Source: three-view drawing plus pictorial views. Frame: mm from the lowest corner of the part. A direction names the side the tool comes from. Round coordinates to 2 decimals unless told otherwise and drop trailing zeros. Loops run counter-clockwise (first coordinate to the right, second up) from the corner with the lowest first, then second, coordinate; pieces in that order, holes last. Notation, with made-up numbers: (-24, 84) -> (22, 84) arc R17 cw to (22, 89) -> close; hole circle Ø10 at (54.25, -39). An arc over 180 degrees is marked (long way). Answer as a JSON object with one key per item and string values. Group by question number.
Item 1: Section query C-C on y = 3.75. Return loops of the section in (x, z), and give its area (3 significant figures).
Item 2: Section query D-D on z = 3. Return loops of the section in (x, y).
Item 3: Section query A-A on x = 2.5. Return loops of the section in (y, z), and give its area (3 significant figures).
Item 4: Pin query (flat end, axial travel): pin 1 (2 mm diameter, centred on y = 1, z = 8, fed in from -X); pin 2 (4 mm diameter, centred on x = 2.5, z = 7, fed in from -Y); pin 3 (0.8 mm diameter, centred on y = 1, z = 6.5, fed in from +X); pin 4 (4 mm diameter, centred on x = 35.5, y = 5, fed in from -Z). Return the tip coordinate at first contact, or that it passes through.
Item 5: Material intervals for line 1 (Z direction, x = 47.5, y = 4.3); line 2 (Z direction, x = 25, y = 3.25); line 3 (X direction, y = 7.25, z = 8), sorted ascending. Write a range as [from, to].
Item 6: Section query B-B on z = 10. Return loops of the section in (x, y).
Item 7: Draft query along Z for the marked faces 1, 2, 3 and 4. Return one class per face: released by +Z, released by -Z, zero draft, split by the parting line, or undercut.
Item 8: Set-up query: the marked faces 5 and 6. Return all of +Z, -Z, +X, -X, +Y, -Y with unobstructed straight access to the full face (end or side cutting, diameter ignored); none if empty.
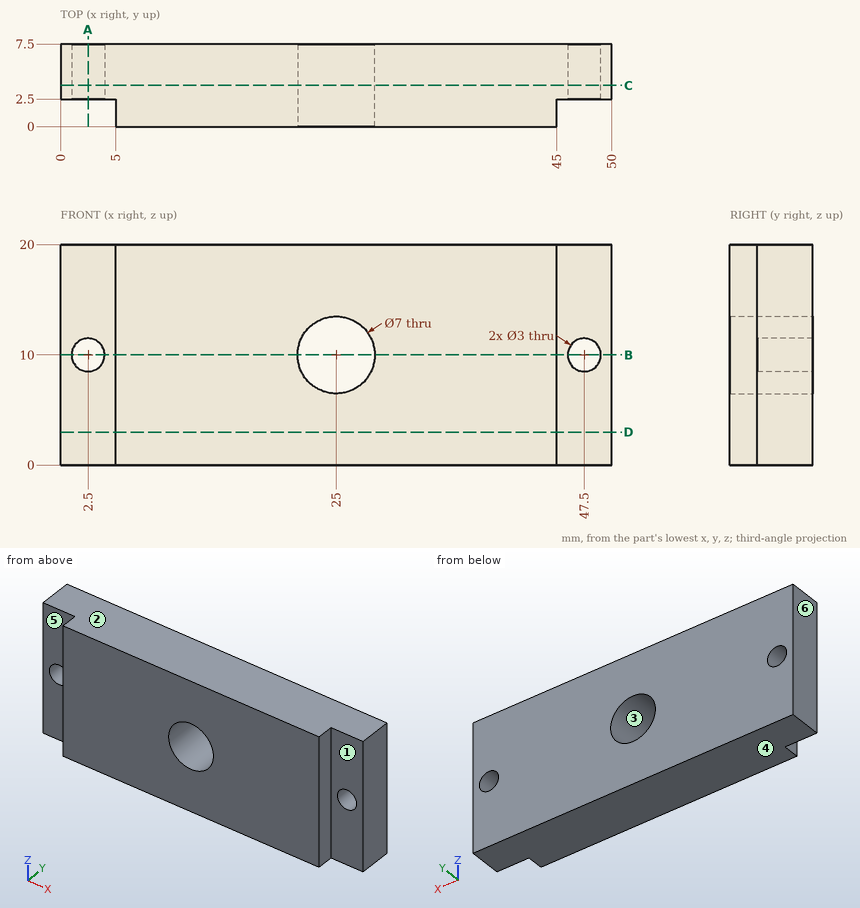
Solved:
{
 "1": {"outline": "(0, 0) -> (50, 0) -> (50, 20) -> (0, 20) -> close; hole circle Ø3 at (2.5, 10); hole circle Ø7 at (25, 10); hole circle Ø3 at (47.5, 10)", "area": "947 mm²"},
 "2": {"outline": "(0, 2.5) -> (5, 2.5) -> (5, 0) -> (45, 0) -> (45, 2.5) -> (50, 2.5) -> (50, 7.5) -> (0, 7.5) -> close"},
 "3": {"outline": "(2.5, 0) -> (7.5, 0) -> (7.5, 8.5) -> (2.5, 8.5) -> close; (2.5, 11.5) -> (7.5, 11.5) -> (7.5, 20) -> (2.5, 20) -> close", "area": "85.0 mm²"},
 "4": {"pin 1": "x = 5", "pin 2": "y = 2.5", "pin 3": "x = 45", "pin 4": "z = 0"},
 "5": {"line 1": "[0, 8.5], [11.5, 20]", "line 2": "[0, 6.5], [13.5, 20]", "line 3": "[0, 22.13], [27.87, 50]"},
 "6": {"outline": "(0, 2.5) -> (1, 2.5) -> (1, 7.5) -> (0, 7.5) -> close; (4, 2.5) -> (5, 2.5) -> (5, 0) -> (21.5, 0) -> (21.5, 7.5) -> (4, 7.5) -> close; (28.5, 0) -> (45, 0) -> (45, 2.5) -> (46, 2.5) -> (46, 7.5) -> (28.5, 7.5) -> close; (49, 2.5) -> (50, 2.5) -> (50, 7.5) -> (49, 7.5) -> close"},
 "7": {"face 1": "zero draft", "face 2": "released by +Z", "face 3": "undercut", "face 4": "released by -Z"},
 "8": {"face 5": "+Z, -Z, -X, -Y", "face 6": "+Z, -Z, -X, +Y, -Y"}
}
